Verification items for the finished model (mm, model axes). Coordinates: 2 decimals unless noted, no trailing zeros. Order: outer loops, then holes, each group sorted by start corner. A loop starts at its lowest first (then second) coordinate and runs counter-clockwise, first axis right, second up. Notation, with made-up numbers: M -10,38.5 L 6,38.5 A14 cw 6,54.5 Z; hole C 86,-32.5 d11. An arc over 180 degrees is marked long. Return JSON: item names as keys, results as strings.
```python
from build123d import *

# Parameters (mm, degrees)
SKETCH006_W     = 12
SKETCH006_H     = 6
PAD002_DEPTH    = 6
SKETCH007_R     = 2.8
POCKET004_DEPTH = 6.001
FILLET_R        = 4


with BuildPart() as part:
    # Sketch006 → Pad002 (new body)
    with BuildSketch(Plane.XZ.offset(5)):
        with Locations((0, 29)):
            Rectangle(SKETCH006_W, SKETCH006_H)
    extrude(amount=PAD002_DEPTH)

    # Sketch007 → Pocket004 (cut, through all)
    with BuildSketch(Plane(origin=(0, -5, 32), x_dir=(-1, 0, 0), z_dir=(0, 0, 1))):
        with Locations((0, 1)):
            Circle(SKETCH007_R)
    extrude(amount=-POCKET004_DEPTH, mode=Mode.SUBTRACT)

    # Fillet
    fillet_edges = [part.edges().sort_by_distance(p)[0] for p in [
        (-6, -11, 29),
        (6, -11, 29),
    ]]
    fillet(fillet_edges, radius=FILLET_R)


solid = part.part
```
Q1. Go/stop test with flat-tipped pins: pin 1 (2 mm diameter, centred on x = -3.5, z = 27.5, fed in from -Y); pin 2 (3 mm diameter, centred on x = 5, z = 28, fed in from -Y); pin 3 (1 mm diameter, centred on y = -8.5, z = 30.5, fed in from +X). Record where each tip stops, or that it passes through.
Values:
{"pin 1": "y = -10.97", "pin 2": "y = -10.71", "pin 3": "x = 5.87"}
Q2. Material ranges on line 1 along X through (y, z) = (-6, 26.6); line 2 along X through (y, z) = (-8.25, 30.7); line 3 along Y through (x, z) = (0, 28.45), recorded low to high.
Values:
{"line 1": "-6 to -2.8, 2.8 to 6", "line 2": "-5.8 to -1.67, 1.67 to 5.8", "line 3": "-11 to -8.8"}
Q3. Cross-section at B-B, the plane z = 30.2. Record the boundary of the cut face in (x, y), and give its area (3 significant figures).
Values:
{"outline": "M -6,-7 A4 ccw -2,-11 L 2,-11 A4 ccw 6,-7 L 6,-5 L 2.62,-5 A2.8 cw long -2.62,-5 L -6,-5 Z", "area": "47.3 mm^2"}
Q4. Cross-section at A-A, the plane y = -6. Record the boundary of the cut face in (x, z).
Values:
{"outline": "M -6,26 L -2.8,26 L -2.8,32 L -6,32 Z; M 2.8,26 L 6,26 L 6,32 L 2.8,32 Z"}
Q5. Cross-section at D-D, the plane y = -7.5. Record the boundary of the cut face in (x, z).
Values:
{"outline": "M -5.97,26 L -2.36,26 L -2.36,32 L -5.97,32 Z; M 2.36,26 L 5.97,26 L 5.97,32 L 2.36,32 Z"}
Q6. Cross-section at C-C, the plane x = 0. Record the boundary of the cut face in (y, z).
Values:
{"outline": "M -11,26 L -8.8,26 L -8.8,32 L -11,32 Z"}
Q7. Draft check along X on faces 1 (the face through (-4.859, -9.797, 29.042)), 2 (the face through (4, -5, 29)), 3 (the face through (-0.1, -8.8, 29)), 4 (the face through (6, -6, 29)). Enter one of: pulls with the +X half, pulls with the -X half, needs draft (parallel to the pull), parting line crosses it, or undercut.
Values:
{"face 1": "pulls with the -X half", "face 2": "needs draft", "face 3": "undercut", "face 4": "pulls with the +X half"}
